Verification items for the finished model (mm, model axes). Round coordinates to 2 decimals unless told otherwise and drop trailing zeros. Write each loop counter-clockwise with the first axis right and the second up, starting at its lowest first coordinate (ties: lowest second). Pieces come first, ordered by that corner, then holes. Notation, with made-up numbers: M 60,51 L 98,51 A14 ccw 98,62 Z; hole C 35.25,37 d6. An arc over 180 degrees is marked long. Write each question's results on one line, items separated by ' | '.
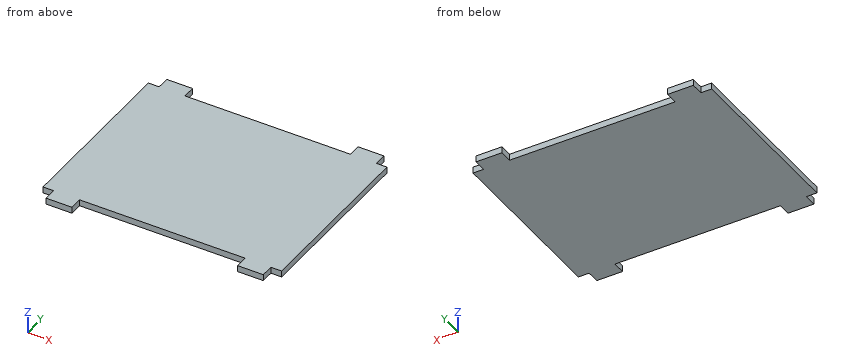
from build123d import *

# Parameters (mm, degrees)
SKETCH1_W           = 60
SKETCH1_H           = 25.35
BOSS_EXTRUDE1_DEPTH = 1.5875
SKETCH2_W           = 41.6
SKETCH2_H           = 3.18
SKETCH2_W_2         = 5.4
CUT_EXTRUDE1_DEPTH  = 1.5875


with BuildPart() as part:
    # Sketch1 → Boss-Extrude1 (new body)
    with BuildSketch(Plane.XY):
        with Locations((0, 12.675)):
            Rectangle(SKETCH1_W, SKETCH1_H)
    boss_extrude1 = extrude(amount=BOSS_EXTRUDE1_DEPTH)

    # Sketch2 → Cut-Extrude1 (cut)
    with BuildSketch(Plane.XY.offset(1.5875)):
        with Locations((0, 23.76)):
            Rectangle(SKETCH2_W, SKETCH2_H)
        with Locations((30, 23.76)):
            Rectangle(SKETCH2_W_2, SKETCH2_H)
        with Locations((-30, 23.76)):
            Rectangle(SKETCH2_W_2, SKETCH2_H)
    cut_extrude1 = extrude(amount=-CUT_EXTRUDE1_DEPTH, mode=Mode.SUBTRACT)

    # Mirror1: Boss-Extrude1, Cut-Extrude1 across plane
    add(boss_extrude1.mirror(Plane.ZX))
    add(cut_extrude1.mirror(Plane.ZX), mode=Mode.SUBTRACT)


solid = part.part
1) Material ranges on line 1 (Y direction, x = -16.5, z = 0.75), recorded low to high. Write a range as [from, to].
Calculated:
line 1: y = [-22.17, 22.17]
2) Depth check by flat-ended pin: P1, Ø0.8, axis at x = -6, z = 0.5, coming from the -Y side; P2, Ø0.5, axis at x = -5, z = 0.5, coming from the +Y side; P3, Ø0.8, axis at y = 23, z = 1, coming from the -X side. Enter the tip coordinate at first touch or a pass-through.
Calculated:
P1: stops at y = -22.17 | P2: stops at y = 22.17 | P3: stops at x = -27.3
3) Sectioned sample at A-A, the plane z = 0.65. Record the cut outline in (x, y).
Calculated:
outline: M -30,-22.17 L -27.3,-22.17 L -27.3,-25.35 L -20.8,-25.35 L -20.8,-22.17 L 20.8,-22.17 L 20.8,-25.35 L 27.3,-25.35 L 27.3,-22.17 L 30,-22.17 L 30,22.17 L 27.3,22.17 L 27.3,25.35 L 20.8,25.35 L 20.8,22.17 L -20.8,22.17 L -20.8,25.35 L -27.3,25.35 L -27.3,22.17 L -30,22.17 Z
4) Sectioned sample at B-B, the plane x = -1. Record the cut outline in (y, z).
Calculated:
outline: M -22.17,0 L 22.17,0 L 22.17,1.59 L -22.17,1.59 Z
